Build history of the part. All positions in model axes, mm. A direction names the side the tool comes from. Coordinates: 2 decimals unless noted, no trailing zeros. Write each loop counter-clockwise with the first axis right and the second up, starting at its lowest first coordinate (ties: lowest second). Pieces come first, ordered by that corner, then holes. Notation, with made-up numbers: (21.5, 74.25) -> (69.5, 74.25) arc R8 ccw to (69.5, 86.25) -> close; hole circle Ø8 at (50.5, 17). An arc over 180 degrees is marked (long way). Write each question's results on one line, items separated by ' | '. Start each with the question number.
Q1. Drop flat-ended pins along their axis: pin 1 Ø5 at (x, z) = (1, 4.5) entering from -Y; pin 2 Ø1.5 at (y, z) = (3.5, 8.5) entering from +X; pin 3 Ø1 at (x, y) = (-11.5, -3.5) entering from -Z; pin 4 Ø2 at (x, y) = (0, 0) entering from -Z. Give the stop position or say it passes through.
Q2. Saw through at B-B on z = 9.5. Give the cut face in (x, y).
Q3. Drill centre lines: line 1 (Y direction, x = 0, z = 12.75); line 2 (Y direction, x = 0, z = 9.5); line 3 (X direction, y = 0, z = 5.75). Where is each one in solid material? Low to high.
Q4. Saw through at A-A on x = 7.75. Give the cut face in (y, z), and give its area (3 significant figures).
Q5. Tool access for faces 1 (the face through (0.27, 1.22, 10.8)), 2 (the face through (-9.27, -2.81, 1.76)), 3 (the face through (2, 2, 12.5)): list every direction of +Z, -Z, +X, -X, +Y, -Y with a clear straight run to the whole face (end or side of a thin tool).
Q6. Saw through at D-D on x = -10.25. Give the cut face in (y, z), and give its area (3 significant figures).
Q7. Two-plate mould, pull along Y, no slides. Class faces 4 (the face through (8.651, 4.624, 1.76)), 5 (the face through (-1, 3, 0)): released by +Y, released by -Y, zero draft, split by the parting line, or undercut.
Q8. Saw through at C-C on z = 17. Give the cut face in (x, y), and give its area (3 significant figures).
from build123d import *

# Parameters (mm, degrees)
F3_D            = 2.5
F3_DEPTH        = 6.5
F3_TIP          = 0.7510757738
F5_DEPTH        = 2.501
F5_COPIES_COUNT = 16


# Not quite as in the source:
# - a pattern or mirror of a feature is missing from the dataset's text; its kind, count and spacing are read off the source's solid


with BuildPart() as f1:
    # F0 (on Front) → F1 (revolve)
    with BuildSketch(Plane.XZ):
        Polygon((-4.5, 0), (-3, 0), (-3, 7.5), (0, 7.5), (0, 19), (-2.5, 19), (-2.5, 12.5), (-4.5, 12.5), (-4.5, 2.5), (-15, 2.5), (-15, 1), (-4.5, 1), align=None)
    revolve(axis=Axis((0, 0, 13.1862424314), (0, 0, 1)))

    # F3
    with Locations(Plane(origin=(0, 0, 7.5), x_dir=(1, 0, 0), z_dir=(0, 0, -1))):
        with Locations((0, 0)):
            Hole(F3_D / 2, depth=F3_DEPTH)
            with Locations((0, 0, -(F3_DEPTH + F3_TIP / 2))):  # 118° drill point
                Cone(0, F3_D / 2, F3_TIP, mode=Mode.SUBTRACT)

    # F4 (on face) → F5 (cut, through all)
    with BuildSketch(Plane.XY.offset(2.5)):
        with BuildLine():
            Line((-1.3722399646, 13.9325861734), (-0.5390942718, 5.4735159967))
            ThreePointArc((-0.5390942718, 5.4735159967), (0, 5.5), (0.5390942718, 5.4735159967))
            Line((0.5390942718, 5.4735159967), (1.3722399646, 13.9325861734))
            ThreePointArc((1.3722399646, 13.9325861734), (0, 14), (-1.3722399646, 13.9325861734))
        make_face()
    f5 = extrude(amount=-F5_DEPTH, mode=Mode.SUBTRACT)

    # F5_copies: F5 ×16 about axis
    f5_copies_axis = Axis((0, 0, 0), (0, 0, 1))
    for i in range(1, F5_COPIES_COUNT):
        add(f5.rotate(f5_copies_axis, i * 360 / F5_COPIES_COUNT), mode=Mode.SUBTRACT)


solid = f1.part
Returned:
1) pin 1: stops at y = -15 | pin 2: stops at x = 3.56 | pin 3: stops at z = 1 | pin 4: stops at z = 14.15
2) outline: circle Ø9 at (0, 0); hole circle Ø2.5 at (0, 0)
3) line 1: y = -2.5 to -1.25, 1.25 to 2.5 | line 2: y = -4.5 to -1.25, 1.25 to 4.5 | line 3: x = -4.5 to -3, 3 to 4.5
4) outline: (-12.84, 1) -> (-9.44, 1) -> (-9.44, 2.5) -> (-12.84, 2.5) -> close; (-6.36, 1) -> (-4.14, 1) -> (-4.14, 2.5) -> (-6.36, 2.5) -> close; (-2.35, 1) -> (-0.76, 1) -> (-0.76, 2.5) -> (-2.35, 2.5) -> close; (0.76, 1) -> (2.35, 1) -> (2.35, 2.5) -> (0.76, 2.5) -> close; (4.14, 1) -> (6.36, 1) -> (6.36, 2.5) -> (4.14, 2.5) -> close; (9.44, 1) -> (12.84, 1) -> (12.84, 2.5) -> (9.44, 2.5) -> close | area: 21.6 mm2
5) face 1: -Z | face 2: +Z, -Z | face 3: +Z
6) outline: (-10.95, 1) -> (-9.54, 1) -> (-9.54, 2.5) -> (-10.95, 2.5) -> close; (-8.41, 1) -> (-5.48, 1) -> (-5.48, 2.5) -> (-8.41, 2.5) -> close; (-3.11, 1) -> (-1.01, 1) -> (-1.01, 2.5) -> (-3.11, 2.5) -> close; (1.01, 1) -> (3.11, 1) -> (3.11, 2.5) -> (1.01, 2.5) -> close; (5.48, 1) -> (8.41, 1) -> (8.41, 2.5) -> (5.48, 2.5) -> close; (9.54, 1) -> (10.95, 1) -> (10.95, 2.5) -> (9.54, 2.5) -> close | area: 19.3 mm2
7) face 4: undercut | face 5: zero draft
8) outline: circle Ø5 at (0, 0) | area: 19.6 mm2
